Source: three-view drawing plus pictorial views. Frame: mm from the lowest corner of the part. A direction names the side the tool comes from. Coordinates: 2 decimals unless noted, no trailing zeros. Write each loop counter-clockwise with the first axis right and the second up, starting at its lowest first coordinate (ties: lowest second). Pieces come first, ordered by that corner, then holes. Notation, with made-up numbers: (68.5, -28) -> (84.5, -28) arc R8 cw to (84.5, -24) -> close; hole circle Ø2 at (32.25, 63.5). An arc over 180 degrees is marked (long way). One line per item, written item: value.
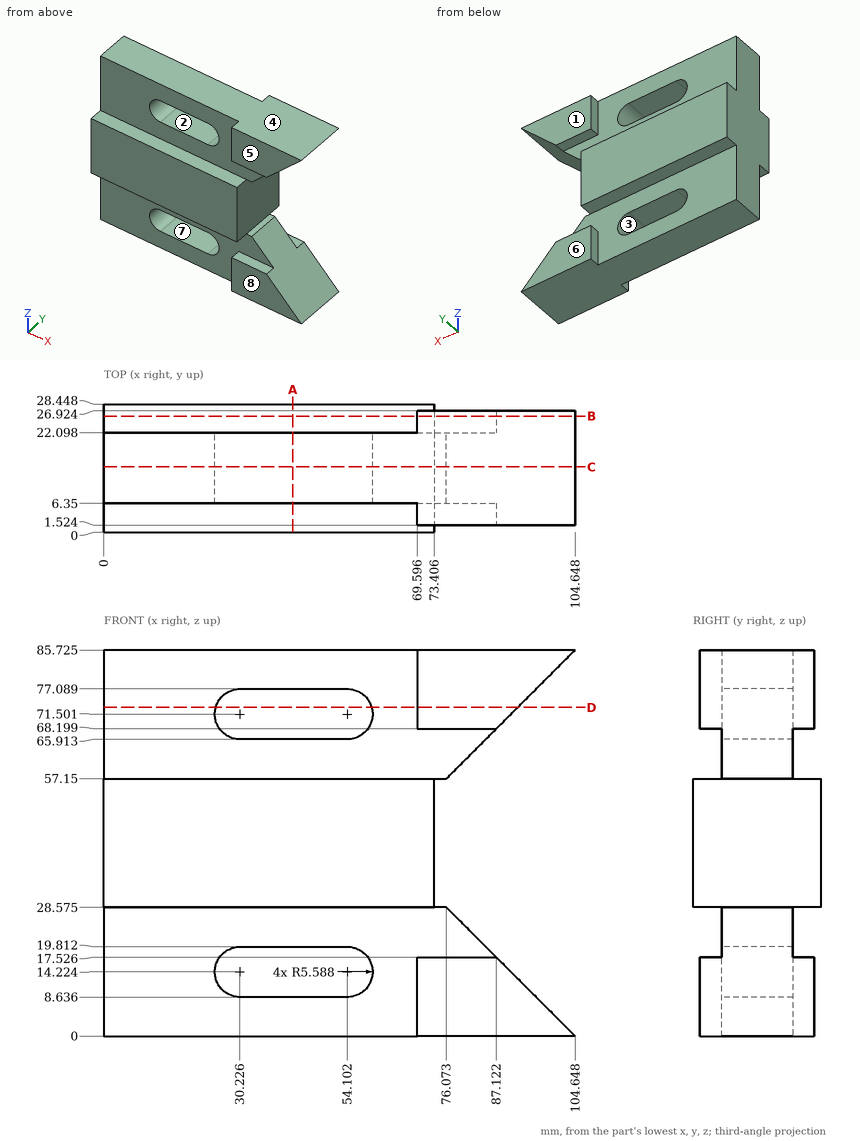
(1) Pull-direction query (Z, two-part tool) for the marked faces 1, 2, 3 and 4; classes: released by +Z, released by -Z, zero draft, split by the parting line, or undercut.
Responses:
face 1: zero draft
face 2: undercut
face 3: undercut
face 4: released by +Z
(2) Line query: line 1 (Z direction, x = 48, y = 13) (3 decimals); line 2 (Z direction, x = 69, y = 3) (3 decimals); line 3 (Y direction, x = 68.5, z = 66.5). Output: solid intervals per line, ascending. Write a range as [from, to].
Responses:
line 1: z = [0, 8.636], [19.812, 65.913], [77.089, 85.725]
line 2: z = [28.575, 57.15]
line 3: y = [6.35, 22.1]
(3) Section D-D (z = 73). Return the cut outline in (x, y), then the cut area to 3 significant figures.
Responses:
outline: (0, 6.35) -> (24.84, 6.35) -> (24.84, 22.1) -> (0, 22.1) -> close; (59.49, 6.35) -> (69.6, 6.35) -> (69.6, 1.52) -> (91.92, 1.52) -> (91.92, 26.92) -> (69.6, 26.92) -> (69.6, 22.1) -> (59.49, 22.1) -> close
area: 1,120 mm2
(4) Section A-A (x = 42). Return the cut outline in (y, z) (3 decimals), then the cut area to 3 significant figures.
Responses:
outline: (0, 28.575) -> (6.35, 28.575) -> (6.35, 19.812) -> (22.098, 19.812) -> (22.098, 28.575) -> (28.448, 28.575) -> (28.448, 57.15) -> (22.098, 57.15) -> (22.098, 65.913) -> (6.35, 65.913) -> (6.35, 57.15) -> (0, 57.15) -> close; (6.35, 0) -> (22.098, 0) -> (22.098, 8.636) -> (6.35, 8.636) -> close; (6.35, 77.089) -> (22.098, 77.089) -> (22.098, 85.725) -> (6.35, 85.725) -> close
area: 1,360 mm2
(5) First-contact query: pin 1 (3 mm diameter, centred on x = 66, z = 69.5, fed in from +Y); pin 2 (14 mm diameter, centred on y = 15, z = 40.5, fed in from +X); pin 3 (9 mm diameter, centred on x = 79.5, z = 10, fed in from +Y). Flat tips, straight axial feed; report the tip coordinate or a pass-through.
Responses:
pin 1: stops at y = 22.1
pin 2: stops at x = 73.41
pin 3: stops at y = 26.92
(6) Reachability of the marked faces 5, 6, 7 and 8 from +Z, -Z, +X, -X, +Y, -Y: full face, straight path, thin tool, end or side. Return the list, or none.
Responses:
face 5: +Z, +X, -X, -Y
face 6: -Z, +X, -X, +Y
face 7: +Y, -Y
face 8: -Z, +X, -X, -Y
(7) Section C-C (y = 14.5). Return the cut outline in (x, z) (3 decimals).
Responses:
outline: (0, 0) -> (104.648, 0) -> (76.073, 28.575) -> (73.406, 28.575) -> (73.406, 57.15) -> (76.073, 57.15) -> (104.648, 85.725) -> (0, 85.725) -> close; hole (30.226, 8.636) -> (54.102, 8.636) arc R5.588 ccw to (54.102, 19.812) -> (30.226, 19.812) arc R5.588 ccw to start; hole (30.226, 65.913) -> (54.102, 65.913) arc R5.588 ccw to (54.102, 77.089) -> (30.226, 77.089) arc R5.588 ccw to start
(8) Section B-B (y = 25.75). Return the cut outline in (x, z) (3 decimals), then the cut area to 3 significant figures.
Responses:
outline: (0, 28.575) -> (73.406, 28.575) -> (73.406, 57.15) -> (0, 57.15) -> close; (69.596, 0) -> (104.648, 0) -> (87.122, 17.526) -> (69.596, 17.526) -> close; (69.596, 68.199) -> (87.122, 68.199) -> (104.648, 85.725) -> (69.596, 85.725) -> close
area: 3,020 mm2
